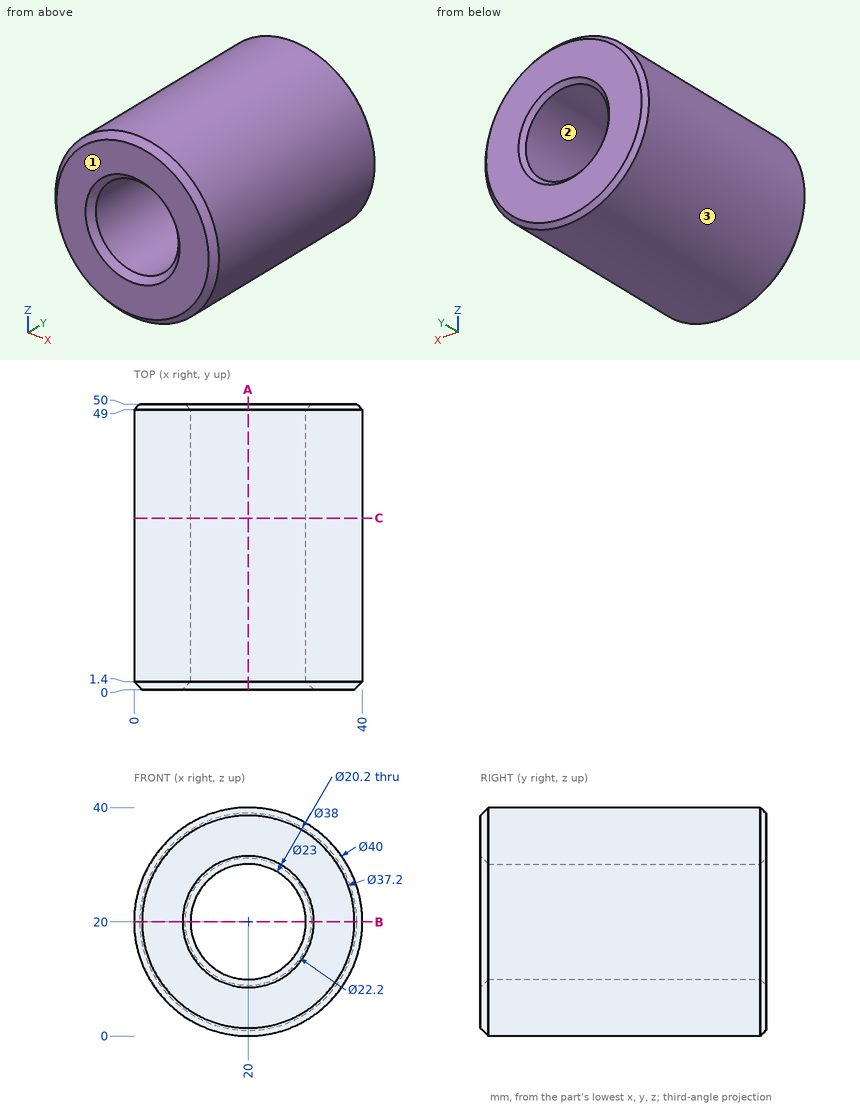
Study the drawing (mm; zero at the part's minimum x, y, z) and answer. Round coordinates to 2 decimals unless told otherwise and drop trailing zeros. Write each loop counter-clockwise with the first axis right and the second up, starting at its lowest first coordinate (ties: lowest second). Pieces come first, ordered by that corner, then holes. Notation, with made-up numbers: (79.25, 13) -> (129.25, 13) arc R17 cw to (129.25, 29) -> close; hole circle Ø7 at (-36.75, 22). An arc over 180 degrees is marked (long way). Answer as CSV lines item,"result". Start each with the question number.
(1) Find the intervals of material crossed by probe 1 along Z at (x, y) = (20, 13); probe 2 along Z at (x, y) = (17, 12.5); probe 3 along X at (y, z) = (37, 16), in increasing order.
(2) The mould has two halves that part along X. Classify the marked faces 1, 2 and 3: +X half, -X half, draft (parallel to the pull), parting line (faces both ways), or undercut.
(3) The part is cut by section A-A, the plane x = 20. Give the vertices of the cut face in (y, z).
(4) The part is cut by section C-C, the plane y = 30. Give the vertices of the cut face in (x, z).
(5) Each of these flat-tipped pins is pushed along its axis until it touches: pin 1 (1.5 mm diameter, centred on y = 15.5, z = 32, fed in from -X); pin 2 (12 mm diameter, centred on x = 25.5, y = 19, fed in from -Z); pin 3 (6 mm diameter, centred on y = 27, z = 35.5, fed in from +X); pin 4 (12 mm diameter, centred on x = 20, z = 20, fed in from -Y). Where does it stop, or does it pass through?
(6) The part is cut by section B-B, the plane z = 20. Give the vertices of the cut face in (x, y), then the cut area to 3 significant figures.
Output values:
1,probe 1,"z = 0 to 9.9, 30.1 to 40"
1,probe 2,"z = 0.23 to 10.36, 29.64 to 39.77"
1,probe 3,"x = 0.4 to 10.73, 29.27 to 39.6"
2,face 1,"draft"
2,face 2,"undercut"
2,face 3,"parting line"
3,outline,"(0, 1.4) -> (1.4, 0) -> (49, 0) -> (50, 1) -> (50, 8.9) -> (49, 9.9) -> (1.4, 9.9) -> (0, 8.5) -> close; (0, 31.5) -> (1.4, 30.1) -> (49, 30.1) -> (50, 31.1) -> (50, 39) -> (49, 40) -> (1.4, 40) -> (0, 38.6) -> close"
4,outline,"circle Ø40 at (20, 20); hole circle Ø20.2 at (20, 20)"
5,pin 1,"stops at x = 3.46"
5,pin 2,"stops at z = 0"
5,pin 3,"stops at x = 35.61"
5,pin 4,"passes through"
6,outline,"(0, 1.4) -> (1.4, 0) -> (8.5, 0) -> (9.9, 1.4) -> (9.9, 49) -> (8.9, 50) -> (1, 50) -> (0, 49) -> close; (30.1, 1.4) -> (31.5, 0) -> (38.6, 0) -> (40, 1.4) -> (40, 49) -> (39, 50) -> (31.1, 50) -> (30.1, 49) -> close"
6,area,"984 mm²"
